Geometry: see drawing. Coordinates: mm, zero at the bounding-box minimum. Give positions to 0.01 mm unless a question says otherwise; leave off trailing zeros. Loops run counter-clockwise (first coordinate to the right, second up) from the corner with the lowest first, then second, coordinate; pieces in that order, holes last. Notation, with made-up numbers: (62, 78.25) -> (75, 78.25) arc R25 ccw to (75, 100.25) -> close; hole circle Ø7 at (59.25, 63.25). An arc over 180 degrees is marked (long way). Use CSV: the item, a comma, the result in double quotes.
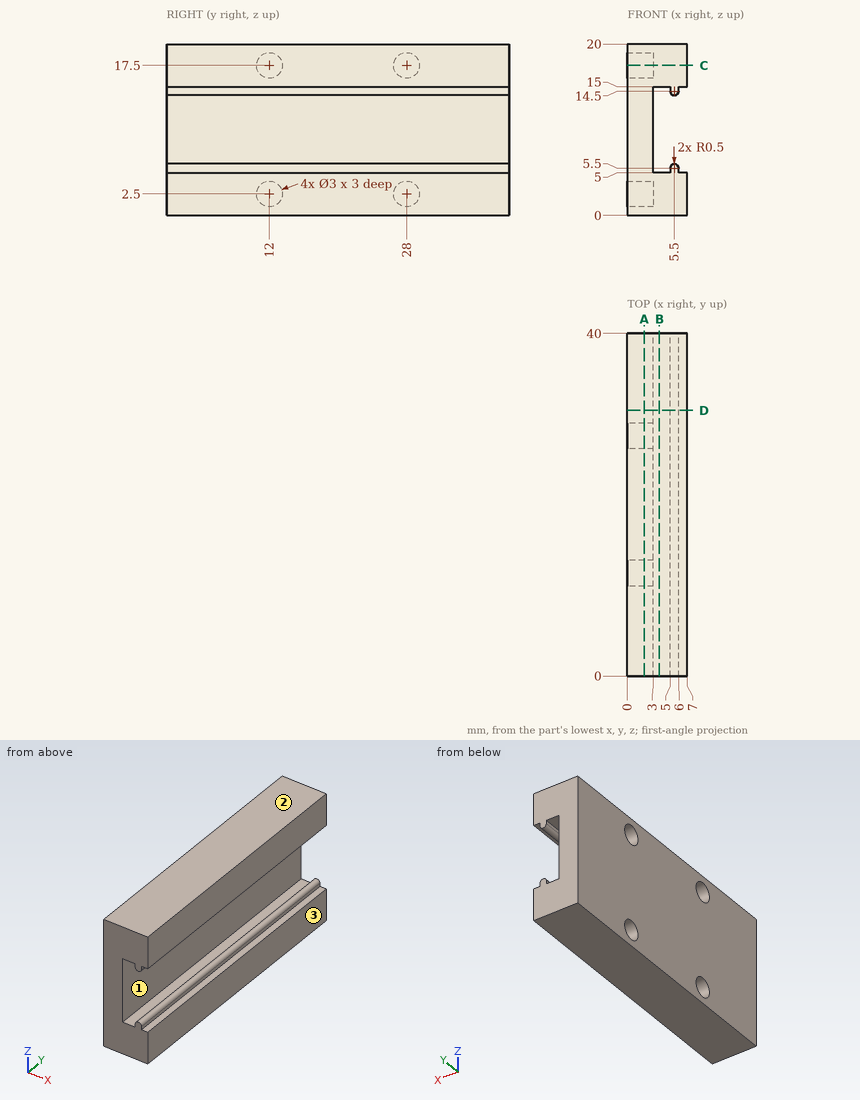
1) Section query D-D (y = 31). Return loops of the section in (x, z), then the cut area to 3 significant figures.
From the geometry:
outline,"(0, 0) -> (7, 0) -> (7, 5) -> (6, 5) -> (6, 5.5) arc R0.5 ccw to (5, 5.5) -> (5, 5) -> (3, 5) -> (3, 15) -> (5, 15) -> (5, 14.5) arc R0.5 ccw to (6, 14.5) -> (6, 15) -> (7, 15) -> (7, 20) -> (0, 20) -> close"
area,"102 mm^2"
2) Section query A-A (x = 2). Return loops of the section in (y, z), then the cut area to 3 significant figures.
From the geometry:
outline,"(0, 0) -> (40, 0) -> (40, 20) -> (0, 20) -> close; hole circle Ø3 at (12, 2.5); hole circle Ø3 at (12, 17.5); hole circle Ø3 at (28, 2.5); hole circle Ø3 at (28, 17.5)"
area,"772 mm^2"
3) Section query B-B (x = 3.75). Return loops of the section in (y, z), then the cut area to 3 significant figures.
From the geometry:
outline,"(0, 0) -> (40, 0) -> (40, 5) -> (0, 5) -> close; (0, 15) -> (40, 15) -> (40, 20) -> (0, 20) -> close"
area,"400 mm^2"
4) Ray query, line 1 (Y direction, x = 2.1, z = 17.5); line 2 (Z direction, x = 3.25, y = 29); line 3 (Z direction, x = 5.25, y = 38). Return the intervals inside material, ascending.
From the geometry:
line 1,"y = 0 to 10.5, 13.5 to 26.5, 29.5 to 40"
line 2,"z = 0 to 5, 15 to 20"
line 3,"z = 0 to 5.93, 14.07 to 20"
5) Mould query, pull axis Z, two halves, no side actions, for the marked faces 1, 2 and 3. Classes: pulls with the +Z half, pulls with the -Z half, needs draft (parallel to the pull), parting line crosses it, or undercut.
From the geometry:
face 1,"undercut"
face 2,"pulls with the +Z half"
face 3,"needs draft"
6) Section query C-C (z = 17.5). Return loops of the section in (x, y).
From the geometry:
outline,"(0, 0) -> (7, 0) -> (7, 40) -> (0, 40) -> (0, 29.5) -> (3, 29.5) -> (3, 26.5) -> (0, 26.5) -> (0, 13.5) -> (3, 13.5) -> (3, 10.5) -> (0, 10.5) -> close"
7) Contact query for flat-ended pins moving along their axis: pin 1 (3 mm diameter, centred on y = 28, z = 10.5, fed in from +X); pin 2 (1.5 mm diameter, centred on y = 27.5, z = 18, fed in from -X). Output: stop coordinate, or through.
From the geometry:
pin 1,"stops at x = 3"
pin 2,"stops at x = 3"
